from build123d import *

# Parameters (mm, degrees)
SKETCH1_R           = 2
BOSS_EXTRUDE1_DEPTH = 8
CHAMFER1_SIZE       = 0.4


with BuildPart() as part:
    # Sketch1 → Boss-Extrude1 (new body)
    with BuildSketch(Plane.XY):
        with BuildLine():
            Line((-66.308814514, -129.547773352), (-43.320112037, -122.388992281))
            ThreePointArc((-43.320112037, -122.388992281), (0, -115.8), (43.320112037, -122.388992281))
            Line((43.320112037, -122.388992281), (66.308814514, -129.547773352))
            ThreePointArc((66.308814514, -129.547773352), (77.091963333, -126.245396489), (77.942286341, -115))
            Line((77.942286341, -115), (61.560254038, -86.62548772))
            ThreePointArc((61.560254038, -86.62548772), (55.488190451, -81.966229458), (47.9, -82.965233683))
            ThreePointArc((47.9, -82.965233683), (0, -95.8), (-47.9, -82.965233683))
            ThreePointArc((-47.9, -82.965233683), (-55.488190451, -81.966229458), (-61.560254038, -86.62548772))
            Line((-61.560254038, -86.62548772), (-77.942286341, -115))
            ThreePointArc((-77.942286341, -115), (-77.091963333, -126.245396489), (-66.308814514, -129.547773352))
        make_face()
        with Locations((-52.9, -91.62548772)):
            Circle(SKETCH1_R, mode=Mode.SUBTRACT)
        with Locations((0, -105.8)):
            Circle(SKETCH1_R, mode=Mode.SUBTRACT)
        with Locations((52.9, -91.62548772)):
            Circle(SKETCH1_R, mode=Mode.SUBTRACT)
        with BuildLine():
            Line((-71.01408311, -119), (-60.632050808, -101.017792566))
            ThreePointArc((-60.632050808, -101.017792566), (-59.41763809, -100.085940913), (-57.9, -100.285741758))
            ThreePointArc((-57.9, -100.285741758), (-50.03884881, -101.207440229), (-43.970129475, -96.126311247))
            ThreePointArc((-43.970129475, -96.126311247), (-42.86414468, -95.145621216), (-41.386723322, -95.192327068))
            ThreePointArc((-41.386723322, -95.192327068), (-26.865416882, -100.263100769), (-11.754209758, -103.132335147))
            ThreePointArc((-11.754209758, -103.132335147), (-10.451372404, -103.830597372), (-9.98390649, -105.23289225))
            ThreePointArc((-9.98390649, -105.23289225), (-9.999586121, -105.709019747), (-9.992572367, -106.185353717))
            ThreePointArc((-9.992572367, -106.185353717), (-10.497515805, -107.592554365), (-11.837059844, -108.256484561))
            ThreePointArc((-11.837059844, -108.256484561), (-28.950552114, -110.551129126), (-45.698686268, -114.750773599))
            Line((-45.698686268, -114.750773599), (-68.687388745, -121.90955467))
            ThreePointArc((-68.687388745, -121.90955467), (-70.844018509, -121.249079298), (-71.01408311, -119))
        make_face(mode=Mode.SUBTRACT)
        with BuildLine():
            Line((71.01408311, -119), (60.632050808, -101.017792566))
            ThreePointArc((60.632050808, -101.017792566), (59.41763809, -100.085940913), (57.9, -100.285741758))
            ThreePointArc((57.9, -100.285741758), (50.03884881, -101.207440229), (43.970129475, -96.126311247))
            ThreePointArc((43.970129475, -96.126311247), (42.86414468, -95.145621216), (41.386723322, -95.192327068))
            ThreePointArc((41.386723322, -95.192327068), (26.865416882, -100.263100769), (11.754209758, -103.132335147))
            ThreePointArc((11.754209758, -103.132335147), (10.451372404, -103.830597372), (9.98390649, -105.23289225))
            ThreePointArc((9.98390649, -105.23289225), (9.999586121, -105.709019747), (9.992572367, -106.185353717))
            ThreePointArc((9.992572367, -106.185353717), (10.497515805, -107.592554365), (11.837059844, -108.256484561))
            ThreePointArc((11.837059844, -108.256484561), (28.950552114, -110.551129126), (45.698686268, -114.750773599))
            Line((45.698686268, -114.750773599), (68.687388745, -121.90955467))
            ThreePointArc((68.687388745, -121.90955467), (70.844018509, -121.249079298), (71.01408311, -119))
        make_face(mode=Mode.SUBTRACT)
    extrude(amount=BOSS_EXTRUDE1_DEPTH)

    # Chamfer1
    chamfer1_edges = [part.edges().sort_by_distance(p)[0] for p in [
        (-69.751270189, -100.81274386, 0),
        (-55.488190451, -81.966229458, 0),
        (0, -95.8, 0),
        (55.488190451, -81.966229458, 0),
        (69.751270189, -100.81274386, 0),
        (77.091963333, -126.245396489, 0),
        (54.814463276, -125.968382816, 0),
        (0, -115.8, 8),
        (0, -115.8, 0),
        (-54.814463276, -125.968382816, 0),
        (-77.091963333, -126.245396489, 0),
        (54.814463276, -125.968382816, 8),
        (77.091963333, -126.245396489, 8),
        (69.751270189, -100.81274386, 8),
        (-54.9, -91.62548772, 0),
        (-54.9, -91.62548772, 8),
        (55.488190451, -81.966229458, 8),
        (-2, -105.8, 0),
        (-2, -105.8, 8),
        (0, -95.8, 8),
        (50.9, -91.62548772, 0),
        (50.9, -91.62548772, 8),
        (-55.488190451, -81.966229458, 8),
        (-69.751270189, -100.81274386, 8),
        (-70.844018509, -121.249079298, 0),
        (-57.193037507, -118.330164135, 0),
        (-28.950552114, -110.551129126, 0),
        (-10.497515805, -107.592554365, 0),
        (-9.999586121, -105.709019747, 0),
        (-10.451372404, -103.830597372, 0),
        (-26.865416882, -100.263100769, 0),
        (-42.86414468, -95.145621216, 0),
        (-50.03884881, -101.207440229, 0),
        (-59.41763809, -100.085940913, 0),
        (-77.091963333, -126.245396489, 8),
        (-65.823066959, -110.008896283, 0),
        (-70.844018509, -121.249079298, 8),
        (-57.193037507, -118.330164135, 8),
        (-28.950552114, -110.551129126, 8),
        (-10.497515805, -107.592554365, 8),
        (-9.999586121, -105.709019747, 8),
        (-10.451372404, -103.830597372, 8),
        (-26.865416882, -100.263100769, 8),
        (-42.86414468, -95.145621216, 8),
        (-50.03884881, -101.207440229, 8),
        (-59.41763809, -100.085940913, 8),
        (-65.823066959, -110.008896283, 8),
        (28.950552114, -110.551129126, 0),
        (57.193037507, -118.330164135, 0),
        (70.844018509, -121.249079298, 0),
        (65.823066959, -110.008896283, 0),
        (59.41763809, -100.085940913, 0),
        (50.03884881, -101.207440229, 0),
        (42.86414468, -95.145621216, 0),
        (26.865416882, -100.263100769, 0),
        (10.451372404, -103.830597372, 0),
        (9.999586121, -105.709019747, 0),
        (10.497515805, -107.592554365, 0),
        (28.950552114, -110.551129126, 8),
        (57.193037507, -118.330164135, 8),
        (70.844018509, -121.249079298, 8),
        (65.823066959, -110.008896283, 8),
        (59.41763809, -100.085940913, 8),
        (50.03884881, -101.207440229, 8),
        (42.86414468, -95.145621216, 8),
        (26.865416882, -100.263100769, 8),
        (10.451372404, -103.830597372, 8),
        (9.999586121, -105.709019747, 8),
        (10.497515805, -107.592554365, 8),
        (-54.814463276, -125.968382816, 8),
    ]]
    chamfer(chamfer1_edges, length=CHAMFER1_SIZE)


solid = part.part
The model under review builds one solid part; all positions refer to its coordinate system, in mm. A direction names the side the tool comes from. Give positions to 0.01 mm unless a question says otherwise; leave off trailing zeros. Write each loop counter-clockwise with the first axis right and the second up, starting at its lowest first coordinate (ties: lowest second). Pieces come first, ordered by that corner, then holes. Notation, with made-up numbers: M 9.25,83 L 52.25,83 A9 ccw 52.25,97 Z; hole C 65,63.25 d4. An arc over 180 degrees is marked long. One line per question, with ' | ' between items. Start each with the question number.
Item 1: For faces 1 (the flat face through (56.97, -118.47, 7.8)), 2 (the flat face through (-55.036, -125.825, 7.803)), 3 (the flat face through (54.654, -125.918, 3.95)), 4 (the flat face through (-66.071, -110.033, 0.197)), list the 3-axis set-ups (+Z, -Z, +X, -X, +Y, -Y) from which the entire face can be reached by the end or side of a thin tool; tool diameter is ignored.
Item 2: We need section A-A on x = 0. Write out the cut boundary in (y, z), plus the area to 3 significant figures.
Item 3: For pin 1 (1.5 mm diameter, centred on x = 40, z = 4.5, fed in from +Y); pin 2 (3.5 mm diameter, centred on x = -52.9, y = -91.63, fed in from +Z); pin 3 (1.5 mm diameter, centred on y = -94.5, z = 7, fed in from +X); pin 4 (4 mm diameter, centred on y = -123.5, z = 5, fed in from -X), all flat-tipped, find the tip position at first contact; note any pin that passes through.
Item 4: Wall thickness on line 1 (Y direction, x = 0, z = 3); line 2 (Y direction, x = 52.9, z = 3); line 3 (Y direction, x = -44.5, z = 6.25): over which ranges is each line inside the solid? List them lowest first. Write a range as from..to.
Item 5: We need section C-C on y = -112. Give the number of separate pieces and of enclosed holes in the cut face, plus the area to 3 significant figures.
Item 6: We need section B-B on x = -52.9. Write out the cut boundary in (y, z), plus the area to 3 significant figures.
Item 7: Draft analysis for pull direction Y (two halves, no side actions). For faces 5 (the flat face through (-1, -100, 8)), 6 (the flat face through (-57.03, -118.28, 3.95)), 7 (the conical face through (-76.96, -125.94, 7.89)), state which applies: released by +Y, released by -Y, zero draft, split by the parting line, or undercut.
Results found:
1) face 1: +Z | face 2: +Z, -Y | face 3: +Z, -Z, -Y | face 4: -Z
2) outline: M -115.8,0.4 L -115.4,0 L -108.2,0 L -107.8,0.4 L -107.8,7.6 L -108.2,8 L -115.4,8 L -115.8,7.6 Z; M -103.8,0.4 L -103.4,0 L -96.2,0 L -95.8,0.4 L -95.8,7.6 L -96.2,8 L -103.4,8 L -103.8,7.6 Z | area: 127 mm2
3) pin 1: stops at y = -86.7 | pin 2: passes through | pin 3: stops at x = 66.54 | pin 4: stops at x = -79.17
4) line 1: y = -115.8..-107.8, -103.8..-95.8 | line 2: y = -125.37..-116.99, -101.63..-93.63, -89.63..-81.63 | line 3: y = -122.76..-114.38, -97.05..-84.84
5) separate pieces: 3 | enclosed holes: 0 | area: 717 mm2
6) outline: M -125.37,0.4 L -124.95,0 L -117.41,0 L -116.99,0.4 L -116.99,7.6 L -117.41,8 L -124.95,8 L -125.37,7.6 Z; M -101.63,0.4 L -101.23,0 L -94.03,0 L -93.63,0.4 L -93.63,7.6 L -94.03,8 L -101.23,8 L -101.63,7.6 Z; M -89.63,0.4 L -89.23,0 L -82.03,0 L -81.63,0.4 L -81.63,7.6 L -82.03,8 L -89.23,8 L -89.63,7.6 Z | area: 194 mm2
7) face 5: zero draft | face 6: undercut | face 7: split by the parting line
